from build123d import *

# Parameters (mm, degrees)
SKETCH1_W           = 50
SKETCH1_H           = 50
BOSS_EXTRUDE1_DEPTH = 50
SKETCH2_W           = 10
SKETCH2_H           = 10
CUT_EXTRUDE1_DEPTH  = 6
FILLET1_R           = 5
FILLET2_R           = 1
SKETCH4_R           = 3
BOSS_EXTRUDE2_DEPTH = 5
CUT_EXTRUDE2_DEPTH  = 4
SKETCH6_W           = 25
SKETCH6_H           = 6
CUT_EXTRUDE3_DEPTH  = 4


with BuildPart() as part:
    # Sketch1 → Boss-Extrude1 (new body)
    with BuildSketch(Plane.XY):
        Rectangle(SKETCH1_W, SKETCH1_H)
    extrude(amount=BOSS_EXTRUDE1_DEPTH)

    # Sketch2 → Cut-Extrude1 (cut)
    with BuildSketch(Plane(origin=(0, 25, 0), x_dir=(1, 0, 0), z_dir=(0, 1, 0))):
        with Locations((-20, -5)):
            Rectangle(SKETCH2_W, SKETCH2_H)
        with Locations((-20, -45)):
            Rectangle(SKETCH2_W, SKETCH2_H)
        with Locations((20, -25)):
            Rectangle(SKETCH2_W, SKETCH2_H)
    extrude(amount=-CUT_EXTRUDE1_DEPTH, mode=Mode.SUBTRACT)

    # Fillet1
    fillet1_edges = [part.edges().sort_by_distance(p)[0] for p in [
        (15, 22, 30),
        (15, 22, 20),
        (-15, 22, 40),
        (-15, 22, 10),
    ]]
    fillet(fillet1_edges, radius=FILLET1_R - 0.0001)  # a hair under: the kernel refuses the full size

    # Fillet2
    fillet2_edges = [part.edges().sort_by_distance(p)[0] for p in [
        (-22.49995, 25, 10),
        (-15, 25, 47.49995),
        (22.49995, 25, 20),
        (22.49995, 25, 30),
        (-22.49995, 25, 40),
        (-15, 25, 2.50005),
        (16.464436805, 25, 28.535563195),
        (16.464436805, 25, 21.464436805),
        (-16.464436805, 25, 41.464436805),
        (-16.464436805, 25, 8.535563195),
    ]]
    fillet(fillet2_edges, radius=FILLET2_R)

    # Sketch4 → Boss-Extrude2 (add)
    with BuildSketch(Plane(origin=(0, 19, 0), x_dir=(1, 0, 0), z_dir=(0, 1, 0))):
        with Locations(Location((-20, -5, 0), (0, 0, 270))):
            Circle(SKETCH4_R)
        with Locations(Location((-20, -45, 0), (0, 0, 90))):
            Circle(SKETCH4_R)
        with Locations(Location((20, -25, 0), (0, 0, 90))):
            Circle(SKETCH4_R)
    extrude(amount=BOSS_EXTRUDE2_DEPTH)

    # Sketch5 → Cut-Extrude2 (cut)
    with BuildSketch(Plane(origin=(0, 24, 0), x_dir=(1, 0, 0), z_dir=(0, 1, 0))):
        Polygon((-20, -3.267949192), (-21.5, -4.133974596), (-21.5, -5.866025404), (-20, -6.732050808), (-18.5, -5.866025404), (-18.5, -4.133974596), align=None)
        Polygon((-20, -43.267949192), (-21.5, -44.133974596), (-21.5, -45.866025404), (-20, -46.732050808), (-18.5, -45.866025404), (-18.5, -44.133974596), align=None)
        Polygon((20, -23.267949192), (18.5, -24.133974596), (18.5, -25.866025404), (20, -26.732050808), (21.5, -25.866025404), (21.5, -24.133974596), align=None)
    extrude(amount=-CUT_EXTRUDE2_DEPTH, mode=Mode.SUBTRACT)

    # Sketch6 → Cut-Extrude3 (cut)
    with BuildSketch(Plane.XY.offset(50)):
        with Locations((0, -16)):
            Rectangle(SKETCH6_W, SKETCH6_H)
    extrude(amount=-CUT_EXTRUDE3_DEPTH, mode=Mode.SUBTRACT)


solid = part.part
Geometry check sheet. Reference: the model listing, model coordinates, mm. A direction names the side the tool comes from. Give positions to 0.01 mm unless a question says otherwise; leave off trailing zeros. Order: outer loops, then holes, each group sorted by start corner. A loop starts at its lowest first (then second) coordinate and runs counter-clockwise, first axis right, second up. Notation, with made-up numbers: (-1, 63) - (53, 63) arc R22 cw to (53, 84) - close; hole circle Ø1 at (22, 14.25). An arc over 180 degrees is marked (long way). Use one line per item in the form item = value.
1) Sectioned sample at A-A (y = -15.5). Record the boundary of the cut face in (x, z), and give its area (3 significant figures).
Working result:
outline = (-25, 0) - (25, 0) - (25, 50) - (12.5, 50) - (12.5, 46) - (-12.5, 46) - (-12.5, 50) - (-25, 50) - close
area = 2,400 mm^2
2) Depth check by flat-ended pin: pin 1 Ø0.9 at (y, z) = (23, 25) entering from +X; pin 2 Ø0.9 at (y, z) = (22.5, 5) entering from -X; pin 3 Ø8 at (x, z) = (-18, 5) entering from +Y; pin 4 Ø1.8 at (x, z) = (-19, 43.5) entering from +Y. Enter the tip coordinate at first touch or a pass-through.
Working result:
pin_1 = 23
pin_2 = -23
pin_3 = 25
pin_4 = 24
3) Access from +Z, -Z, +X, -X, +Y, -Y to the whole of each face (thin tool, end or side, straight path). Record for faces 1 (the face through (22, 22, 20)), 2 (the face through (-25, 0, 25)), 3 (the face through (-21.3, 24, 6.3)), 4 (the face through (-20.76, 22.028, 46.293)).
Working result:
face_1 = +X, +Y
face_2 = +Z, -Z, -X, +Y, -Y
face_3 = -Z, -X, +Y
face_4 = +Y
4) Material ranges on probe 1 along Z at (x, y) = (0.5, -17); probe 2 along Y at (x, z) = (-11, 47.5); probe 3 along X at (y, z) = (19.5, 21), recorded low to high. Write a range as from..to.
Working result:
probe_1 = 0..46
probe_2 = -25..-19, -13..25
probe_3 = -25..17
5) Draft check along Y on faces 5 (the face through (-18.7, 24, 43.7)), 6 (the face through (-12.5, -16, 48)), 7 (the face through (0, 0, 50)), 8 (the face through (12.5, -16, 48)). Enter one of: released by +Y, released by -Y, zero draft, split by the parting line, or undercut.
Working result:
face_5 = released by +Y
face_6 = undercut
face_7 = zero draft
face_8 = undercut
